Autodesk Inventor part; units mm, degrees
ref_plane "YZ Plane" through (0, 0, 0) normal (1, 0, 0) x (0, 1, 0)
ref_plane "XZ Plane" through (0, 0, 0) normal (0, 1, 0) x (-1, 0, 0)
ref_plane "XY Plane" through (0, 0, 0) normal (0, 0, 1) x (1, 0, 0)
sketch "Sketch1" plane through (0, 0, 0) normal (0, 0, 1) x (1, 0, 0)
  line L0 (0, 0) -> (0, 30)
  line L1 (0, 30) -> (-6.5, 30)
  line L2 (0, 0) -> (-45, 0)
  line L3 (-45, 0) -> (-45, -11.8)
  line L4 (-45, -11.8) -> (-67.5, -11.8)
  line L5 (-67.5, -11.8) -> (-67.5, 31.8)
  line L6 (-67.5, 31.8) -> (-45, 31.8)
  line L7 (-45, 31.8) -> (-45, 20)
  line L8 (-45, 20) -> (-16.5, 20)
  arc A0 (-16.5, 20) -> (-6.5, 30) centre (-32.1155, 45.6155) ccw
  line L9 (-135, 0) -> (-135, 30)
  line L10 (-135, 30) -> (-128.5, 30)
  line L11 (-135, 0) -> (-90, 0)
  line L12 (-90, 0) -> (-90, -11.8)
  line L13 (-90, -11.8) -> (-67.5, -11.8)
  line L14 (-67.5, 31.8) -> (-90, 31.8)
  line L15 (-90, 31.8) -> (-90, 20)
  line L16 (-90, 20) -> (-118.5, 20)
  arc A1 (-128.5, 30) -> (-118.5, 20) centre (-102.8845, 45.6155) ccw
  dimension "d16" = 10
  dimension "d17" = 30
  dimension "d18" = 6.5
  dimension "d19" = 10
  dimension "d20" = 20
  dimension "d23" = 45
  dimension "d24" = 135
  dimension "d25" = 43.6
extrude "Body" add sketch "Sketch1" along normal blind 3
sketch "Sketch2" plane through (0, 0, 3) normal (0, 0, 1) x (1, 0, 0)
  line L0 (-72.5, -4.3) -> (-72.5, 24.3)
  arc A0 (-62.5, 24.3) -> (-72.5, 24.3) centre (-67.5, 24.3) ccw
  line L1 (-62.5, 24.3) -> (-62.5, -4.3)
  arc A1 (-72.5, -4.3) -> (-62.5, -4.3) centre (-67.5, -4.3) ccw
  line L2 (-16.5, 20) -> (-45, 20)
  line L3 (0, 0) -> (0, 30)
  line L4 (-45, -11.8) -> (-45, 0)
  line L5 (-45, 20) -> (-45, 0)
  line L6 (-131.212, 10) -> (6.3115, 10)
  point P0 (-62.5, 10)
  point P1 (-45, 10)
  dimension "d28" = 28.6
  dimension "d30" = 62.5
  dimension "d31" = 10
extrude "Extrusion2" cut sketch "Sketch2" against normal through all
draft "FaceDraft1" angle -20 pull direction (0, 0, 1) faces at (0, 10, 1) fixed edges at (0, 15, 3)
draft "FaceDraft2" angle -20 pull direction (0, 0, 1) faces at (-135, 20, 1) fixed edges at (-135, 15, 3)
equation "\"d16\" = deslizador_interruptor_largo"
equation "\"d17\" = deslizador_interruptor_angulo"
equation "\"d18\" = deslizador_interruptor_separacion"
equation "\"d19\" = deslizador_interruptor_ancho"
equation "\"d20\" = deslizador_ancho"
equation "\"d23\" = deslizador_apoyo_largo"
equation "\"d24\" = deslizador_largo"
equation "\"d25\" = deslizador_ancho + 2 * deslizador_apoyo_ancho"
equation "\"d26\" = deslizador_grosor"
equation "\"d28\" = deslizador_eje_movimiento"
equation "\"d30\" = deslizador_eje_separacion"
equation "\"d31\" = deslizador_eje_ancho"
equation "\"d34\" = tirador_deslizador_agarre"
equation "\"d35\" = tirador_deslizador_agarre"
properties part number "Deslizador"
Geometry: final body of the model. Coordinates: model frame, mm. A direction names the side the tool comes from. Give positions to 0.01 mm unless a question says otherwise; leave off trailing zeros. Order: outer loops, then holes, each group sorted by start corner. A loop starts at its lowest first (then second) coordinate and runs counter-clockwise, first axis right, second up. Notation, with made-up numbers: (14.5, 55.25) -> (34.5, 55.25) arc R19 cw to (34.5, 68.25) -> close; hole circle Ø1 at (-14, -15). An arc over 180 degrees is marked (long way). Answer as a JSON object with one key per item and string values.
Q1. Access query for faces 4 (the cylindrical face through (-10.832, 24.473, 1.479)), 5 (the flat face through (-132, 30, 1)), 6 (the flat face through (-113, 0, 1)), 7 (the flat face through (-45, -6, 1)), 8 (the cylindrical face through (-67.6, -9.3, 1.5)). Directions: +Z, -Z, +X, -X, +Y, -Y. A direction counts if a zero-diameter tool reaches every point of the face in a straight line with its end or side. Return the directions, or none.
Entries:
{"face 4": "+Z, -Z, +Y", "face 5": "+Z, -Z, -X, +Y", "face 6": "+Z, -Z, -X, -Y", "face 7": "+Z, -Z, +X, -Y", "face 8": "+Z, -Z"}
Q2. Section A-A (x = -67.5). Output: boundary loops of the cut face in (y, z), plus the area to 3 significant figures.
Entries:
{"outline": "(-11.8, 0) -> (-9.3, 0) -> (-9.3, 3) -> (-11.8, 3) -> close; (29.3, 0) -> (31.8, 0) -> (31.8, 3) -> (29.3, 3) -> close", "area": "15.0 mm^2"}
Q3. Section D-D (x = -40.5). Output: boundary loops of the cut face in (y, z).
Entries:
{"outline": "(0, 0) -> (20, 0) -> (20, 3) -> (0, 3) -> close"}
Q4. Section C-C (z = 2.4). Output: boundary loops of the cut face in (x, y), plus the area to 3 significant figures.
Entries:
{"outline": "(-134.78, 0) -> (-90, 0) -> (-90, -11.8) -> (-45, -11.8) -> (-45, 0) -> (-0.22, 0) -> (-0.22, 30) -> (-6.5, 30) arc R30 cw to (-16.5, 20) -> (-45, 20) -> (-45, 31.8) -> (-90, 31.8) -> (-90, 20) -> (-118.5, 20) arc R30 cw to (-128.5, 30) -> (-134.78, 30) -> close; hole (-72.5, -4.3) arc R5 ccw to (-62.5, -4.3) -> (-62.5, 24.3) arc R5 ccw to (-72.5, 24.3) -> close", "area": "3,600 mm^2"}
Q5. Draft query along Y for faces 1 (the flat face through (-90, -6, 1)), 2 (the flat face through (-31, 20, 1)), 3 (the cylindrical face through (-67.4, 29.3, 1.5)). Return one class per face: released by +Y, released by -Y, zero draft, split by the parting line, or undercut.
Entries:
{"face 1": "zero draft", "face 2": "released by +Y", "face 3": "undercut"}
Q6. Material intervals for probe 1 along X at (y, z) = (27.5, 2.6); probe 2 along X at (y, z) = (28, 2.25); probe 3 along X at (y, z) = (-3, 0.2), sorted ascending.
Entries:
{"probe 1": "x = -134.85 to -126.8, -90 to -71.34, -63.66 to -45, -8.2 to -0.15", "probe 2": "x = -134.73 to -127.17, -90 to -70.86, -64.14 to -45, -7.83 to -0.27", "probe 3": "x = -90 to -72.5, -62.5 to -45"}
Q7. First-contact query: pin 1 (0.9 mm diameter, centred on y = 12.5, z = 1.5, fed in from +X); pin 2 (1.5 mm diameter, centred on x = -44, z = 0.5, fed in from +Y); pin 3 (1.5 mm diameter, centred on y = 24, z = 1.5, fed in from +X). Flat tips, straight axial feed; report the tip coordinate or a pass-through.
Entries:
{"pin 1": "stops at x = -0.38", "pin 2": "stops at y = 20", "pin 3": "stops at x = -0.27"}
Q8. Section B-B (y = 7). Output: boundary loops of the cut face in (x, z), plus the area to 3 significant figures.
Entries:
{"outline": "(-135, 3) -> (-133.91, 0) -> (-72.5, 0) -> (-72.5, 3) -> close; (-62.5, 0) -> (-1.09, 0) -> (0, 3) -> (-62.5, 3) -> close", "area": "372 mm^2"}
